Work out the finished part from the listing and answer in its coordinate system (mm). A direction names the side the tool comes from. Round coordinates to 2 decimals unless told otherwise and drop trailing zeros. Loops run counter-clockwise (first coordinate to the right, second up) from the corner with the lowest first, then second, coordinate; pieces in that order, holes last.
```python
from build123d import *

# Parameters (mm, degrees)
BOSS_EXTRUDE1_DEPTH = 50
SKETCH3_W           = 6
SKETCH3_H           = 10
CUT_EXTRUDE1_DEPTH  = 18


with BuildPart() as part:
    # Sketch2 → Boss-Extrude1 (new body)
    with BuildSketch(Plane(origin=(0, 0, 0), x_dir=(1, 0, 0), z_dir=(0, 1, 0))):
        with BuildLine():
            Line((29.68807717, 23.68807717), (23.68807717, 23.68807717))
            ThreePointArc((23.68807717, 23.68807717), (30.949964339, 12.819894984), (33.5, 0))
            ThreePointArc((33.5, 0), (30.949964339, -12.819894984), (23.68807717, -23.68807717))
            Line((23.68807717, -23.68807717), (33.68807717, -23.68807717))
            add(Edge.make_bspline(
                [(29.68807717, 23.68807717), (47.221735333, 1.183613852), (33.68807717, -23.68807717)],
                knots=[0, 0, 0, 1, 1, 1], degree=2))
        make_face()
    extrude(amount=BOSS_EXTRUDE1_DEPTH)

    # Sketch3 → Cut-Extrude1 (cut)
    with BuildSketch(Plane.XY.offset(23.68807717)):
        with Locations((36.68807717, 12.5)):
            Rectangle(SKETCH3_W, SKETCH3_H)
    extrude(amount=-CUT_EXTRUDE1_DEPTH, mode=Mode.SUBTRACT)


solid = part.part
```
1. Find section A-A (x = 28.25). Write down the section's boundary in (y, z).
Answer key:
outline: (0, -23.69) - (50, -23.69) - (50, -18.01) - (0, -18.01) - close; (0, 18.01) - (50, 18.01) - (50, 23.69) - (0, 23.69) - close
2. Which of the six approach directions +Z, -Z, +X, -X, +Y, -Y give full straight-line access (tool end or side, diameter ignored) to faces 4 (the face through (36, 7.5, 13)), 5 (the face through (34, 50, 3))?
Answer key:
face 4: +Z, +X
face 5: +Z, -Z, +X, -X, +Y
3. Determine the mould class of faces 1 (the face through (34, 0, 3)), 2 (the face through (37, 13, 5.688)), 3 (the face through (29, 25, 23.688)) for opening direction Y: +Y half, -Y half, draft (parallel to the pull), parting line (faces both ways), or undercut.
Answer key:
face 1: -Y half
face 2: undercut
face 3: draft
4. Consider probe 1 along Y at (x, z) = (34.5, 8); probe 2 along Z at (x, y) = (25.75, 15); probe 3 along Z at (x, y) = (28.25, 44). Determine where each line is inside the solid, lowest interval first.
Answer key:
probe 1: y = 0 to 7.5, 17.5 to 50
probe 2: z = -23.69 to -21.43, 21.43 to 23.69
probe 3: z = -23.69 to -18.01, 18.01 to 23.69
5. Given pin 1 (8 mm diameter, centred on x = 34, y = 44.5, fed in from +Z); pin 2 (4 mm diameter, centred on y = 22, z = -8.5, fed in from +X); pin 3 (1.5 mm diameter, centred on y = 39.5, z = -8, fed in from +X); pin 4 (4 mm diameter, centred on x = 33, y = 20.5, fed in from -Z), each flat-ended and moving along its own axis, determine where each tip first touches the part or whether it passes through.
Answer key:
pin 1: stops at z = 23.69
pin 2: stops at x = 38.46
pin 3: stops at x = 38.27
pin 4: stops at z = -21.94
